Build history of the part. All positions in model axes, mm. A direction names the side the tool comes from. Round coordinates to 2 decimals unless told otherwise and drop trailing zeros. Write each loop counter-clockwise with the first axis right and the second up, starting at its lowest first coordinate (ties: lowest second). Pieces come first, ordered by that corner, then holes. Notation, with made-up numbers: (2.5, 39) -> (7.5, 39) arc R11 ccw to (7.5, 56) -> close; hole circle Ø10 at (-27.75, 71.5). An arc over 180 degrees is marked (long way). Answer as CSV lines item,"result".
Autodesk Inventor part; units mm, degrees
ref_plane "YZ Plane" through (0, 0, 0) normal (1, 0, 0) x (0, 1, 0)
ref_plane "XZ Plane" through (0, 0, 0) normal (0, 1, 0) x (-1, 0, 0)
ref_plane "XY Plane" through (0, 0, 0) normal (0, 0, 1) x (1, 0, 0)
sketch "スケッチ1" plane through (0, 0, 0) normal (0, 0, 1) x (1, 0, 0)
  circle A0 centre (0, 0) radius 10.5 construction
  circle A1 centre (-13.5, 1) radius 1.35
  line L0 (-13.5, 28) -> (13.5, 28) construction
  line L1 (13.5, 28) -> (13.5, 1) construction
  line L2 (13.5, 1) -> (-13.5, 1) construction
  line L3 (-13.5, 1) -> (-13.5, 28) construction
  circle A2 centre (-13.5, 28) radius 1.35
  circle A3 centre (13.5, 1) radius 1.35
  circle A4 centre (13.5, 28) radius 1.35
  line L4 (-19.75, 30.5) -> (-19.75, 27.6)
  line L5 (-19.75, 30.5) -> (19.75, 30.5)
  line L6 (19.75, 30.5) -> (19.75, 27.6)
  line L7 (-19.75, 1.4) -> (-19.75, -1.5)
  line L8 (-19.75, -1.5) -> (-10.6448, -1.5)
  line L9 (19.75, 1.4) -> (19.75, -1.5)
  line L10 (19.75, -1.5) -> (10.6448, -1.5)
  line L11 (-19.75, 25.5) -> (-21.75, 25.5)
  line L12 (-21.75, 25.5) -> (-21.75, 3.5)
  line L13 (-21.75, 3.5) -> (-19.75, 3.5)
  arc A5 (-19.75, 25.5) -> (-19.75, 27.6) centre (-19.75, 26.55) ccw
  arc A6 (-19.75, 1.4) -> (-19.75, 3.5) centre (-19.75, 2.45) ccw
  line L14 (19.75, 25.5) -> (21.75, 25.5)
  line L15 (21.75, 25.5) -> (21.75, 3.5)
  line L16 (21.75, 3.5) -> (19.75, 3.5)
  arc A7 (19.75, 27.6) -> (19.75, 25.5) centre (19.75, 26.55) ccw
  line L17 (0, 28) -> (0, 0) construction
  arc A8 (19.75, 3.5) -> (19.75, 1.4) centre (19.75, 2.45) ccw
  line L18 (-13.5, 14.5) -> (-21.75, 14.5) construction
  arc A9 (10.6448, -1.5) -> (-10.6448, -1.5) centre (0, 0) ccw
  point P0 (0, 30.5)
  dimension "d8" = 21
  dimension "d10" = 27
  dimension "d12" = 1
  dimension "d13" = 2.7
  dimension "d38" = 27
  dimension "d44" = 27
  dimension "d47" = 1.05
  dimension "d48" = 39.5
  dimension "d49" = 2
  dimension "d50" = 5
  dimension "d51" = 32
  dimension "d52" = 5
  dimension "d53" = 10.75
extrude "押し出し1" add sketch "スケッチ1" along normal blind 2
fillet "フィレット1" radius 2 2 edges at (-10.6448, -1.5, 1) (10.6448, -1.5, 1)
sketch "スケッチ3" plane through (0, 0, 2) normal (0, 0, 1) x (1, 0, 0)
  circle A0 centre (-13.5, 1) radius 1.35
  circle A1 centre (-13.5, 1) radius 1.35
  circle A2 centre (13.5, 1) radius 1.35
  circle A3 centre (13.5, 1) radius 1.35
  circle A4 centre (13.5, 28) radius 1.35
  circle A5 centre (13.5, 28) radius 1.35
  circle A6 centre (-13.5, 28) radius 1.35
  circle A7 centre (-13.5, 28) radius 1.35
  point P0 (0, 0)
extrude "押し出し3" add sketch "スケッチ3" against normal up to surface (2 mm away)
equation "\"d38\" = d10"
equation "\"d44\" = d10"
equation "\"d50\" = d30"
equation "\"d51\" = d18 + 2 * d30"
equation "\"d52\" = d50"
properties part number "足首_サブフレーム_1_1" material "アルミニウム 2014-T4"
1. Mould opens along X. For faces 6 (the flat face through (-21, 25.5, 1)), 7 (the cylindrical face through (-11.369, -0.956, 1.014)), 8 (the cylindrical face through (11.34, -0.93, 1.01)), 9 (the flat face through (19.75, 29, 1)) say: +X half, -X half, draft (parallel to the pull), parting line (faces both ways), or undercut.
Results found:
face 6,"draft"
face 7,"undercut"
face 8,"undercut"
face 9,"+X half"
2. Cut at C-C, the plane y = 26.55. Write the cut outline in (x, z).
Results found:
outline,"(-18.7, 0) -> (18.7, 0) -> (18.7, 2) -> (-18.7, 2) -> close"
3. Cut at A-A, the plane y = 2.45. Write the cut outline in (x, z).
Results found:
outline,"(-18.7, 0) -> (-10.47, 0) -> (-10.47, 2) -> (-18.7, 2) -> close; (10.47, 0) -> (18.7, 0) -> (18.7, 2) -> (10.47, 2) -> close"
4. Probe line 1 along X through (y, z) = (5, 1.65); line 2 along Y through (x, z) = (19, 0.7); line 3 along X through (y, z) = (9, 0.25). List the from-to ranges inside material, lowest first.
Results found:
line 1,"x = -21.75 to -9.52, 9.52 to 21.75"
line 2,"y = -1.5 to 1.72, 3.18 to 25.82, 27.28 to 30.5"
line 3,"x = -21.75 to -5.88, 5.88 to 21.75"
5. Which spindle directions (+Z, -Z, +X, -X, +Y, -Y) get a long thin tool onto all of the face, cutting with end or side? Do faces 1 (the flat face through (-21, 3.5, 1)), 2 (the flat face through (19.75, 0, 1)), 3 (the flat face through (-19.75, 29, 1)), 4 (the flat face through (0, 18, 2)), 5 (the flat face through (21, 25.5, 1)). Say none if no direction does.
Results found:
face 1,"+Z, -Z, -X, -Y"
face 2,"+Z, -Z, +X, -Y"
face 3,"+Z, -Z, -X, +Y"
face 4,"+Z, +X, -X, +Y, -Y"
face 5,"+Z, -Z, +X, +Y"
6. Cut at B-B, the plane z = 0.3. Write the cut outline in (x, y), then the cut area to 3 significant figures.
Results found:
outline,"(-21.75, 3.5) -> (-19.75, 3.5) arc R1.05 cw to (-19.75, 1.4) -> (-19.75, -1.5) -> (-12.74, -1.5) arc R2 ccw to (-10.74, 0.42) arc R10.75 cw to (10.74, 0.42) arc R2 ccw to (12.74, -1.5) -> (19.75, -1.5) -> (19.75, 1.4) arc R1.05 cw to (19.75, 3.5) -> (21.75, 3.5) -> (21.75, 25.5) -> (19.75, 25.5) arc R1.05 cw to (19.75, 27.6) -> (19.75, 30.5) -> (-19.75, 30.5) -> (-19.75, 27.6) arc R1.05 cw to (-19.75, 25.5) -> (-21.75, 25.5) -> close"
area,"1,130 mm2"
7. Cut at D-D, the plane x = 3.5. Write the cut outline in (y, z).
Results found:
outline,"(10.16, 0) -> (30.5, 0) -> (30.5, 2) -> (10.16, 2) -> close"
8. Drop flat-ended pins along their axis: pin 1 Ø0.6 at (x, z) = (-20.5, 1.5) entering from -Y; pin 2 Ø0.6 at (x, z) = (20.5, 1) entering from +Y; pin 3 Ø1 at (y, z) = (29.5, 1.5) entering from -X. Give the stop position or say it passes through.
Results found:
pin 1,"stops at y = 3.5"
pin 2,"stops at y = 25.5"
pin 3,"stops at x = -19.75"
